```python
from build123d import *

# Parameters (mm, degrees)
ESQUISSE1_W        = 173
ESQUISSE1_H        = 273
ESQUISSE1_R        = 1.5
ESQUISSE1_W_2      = 87
ESQUISSE1_H_2      = 182
BOSS_EXTRU_1_DEPTH = 4
CONG_1_R           = 3
D_GAGEMENT_M31_D   = 3.4


with BuildPart() as part:
    # Esquisse1 → Boss.-Extru.1 (new body)
    with BuildSketch(Plane.XY):
        with Locations((86.5, 136.5)):
            Rectangle(ESQUISSE1_W, ESQUISSE1_H)
        with Locations((7.62, 236.5)):
            Circle(ESQUISSE1_R, mode=Mode.SUBTRACT)
        with Locations((7.62, 70.5)):
            Circle(ESQUISSE1_R, mode=Mode.SUBTRACT)
        with Locations((158, 236.5)):
            Circle(ESQUISSE1_R, mode=Mode.SUBTRACT)
        with Locations((86.5, 123)):
            Rectangle(ESQUISSE1_W_2, ESQUISSE1_H_2, mode=Mode.SUBTRACT)
    extrude(amount=BOSS_EXTRU_1_DEPTH)

    # Congé1
    cong_1_edges = [part.edges().sort_by_distance(p)[0] for p in [
        (43, 214, 2),
        (43, 32, 2),
        (130, 32, 2),
        (130, 214, 2),
        (0, 273, 2),
        (173, 273, 2),
        (173, 0, 2),
        (0, 0, 2),
    ]]
    fillet(cong_1_edges, radius=CONG_1_R)

    # Dégagement M31 (through all)
    with Locations(Plane.XY.offset(4)):
        with Locations((7.62, 236.5), (7.62, 70.5), (158, 236.5)):
            Hole(D_GAGEMENT_M31_D / 2)


solid = part.part
```
Source: CAD feature listing. Evaluate the final solid. Frame: model axes, mm. Coordinates: 2 decimals unless noted, no trailing zeros. Write each loop counter-clockwise with the first axis right and the second up, starting at its lowest first coordinate (ties: lowest second). Pieces come first, ordered by that corner, then holes. Notation, with made-up numbers: (-5, 18) -> (52, 18) arc R16 ccw to (52, 33) -> close; hole circle Ø10 at (47, 48.25). An arc over 180 degrees is marked (long way). Return JSON: item names as keys, results as strings. Group by question number.
1) Section query A-A, the plane y = 42. Return loops of the section in (x, z).
2) Ray query, line 1 along Y through (x, z) = (7.62, 2.85); line 2 along X through (y, z) = (236.5, 2.5); line 3 along X through (y, z) = (103, 0.8). Return the intervals inside material, ascending.
3) Section query B-B, the plane x = 111.5. Return loops of the section in (y, z), plus the area to 3 significant figures.
From the geometry:
{
 "1": {"outline": "(0, 0) -> (43, 0) -> (43, 4) -> (0, 4) -> close; (130, 0) -> (173, 0) -> (173, 4) -> (130, 4) -> close"},
 "2": {"line 1": "0 to 68.8, 72.2 to 234.8, 238.2 to 273", "line 2": "0 to 5.92, 9.32 to 156.3, 159.7 to 173", "line 3": "0 to 43, 130 to 173"},
 "3": {"outline": "(0, 0) -> (32, 0) -> (32, 4) -> (0, 4) -> close; (214, 0) -> (273, 0) -> (273, 4) -> (214, 4) -> close", "area": "364 mm²"}
}
